Model file for the job. Use its own axes, mm. Face numbers are marked on the shaded views. Round coordinates to 2 decimals unless told otherwise and drop trailing zeros. Order: outer loops, then holes, each group sorted by start corner. A loop starts at its lowest first (then second) coordinate and runs counter-clockwise, first axis right, second up. Notation, with made-up numbers: (-30.5, 59.25) - (-9.5, 59.25) arc R12 ccw to (-9.5, 63.25) - close; hole circle Ø2 at (81.25, 63.5). An arc over 180 degrees is marked (long way). Write item = value, one per line. Start each with the question number.
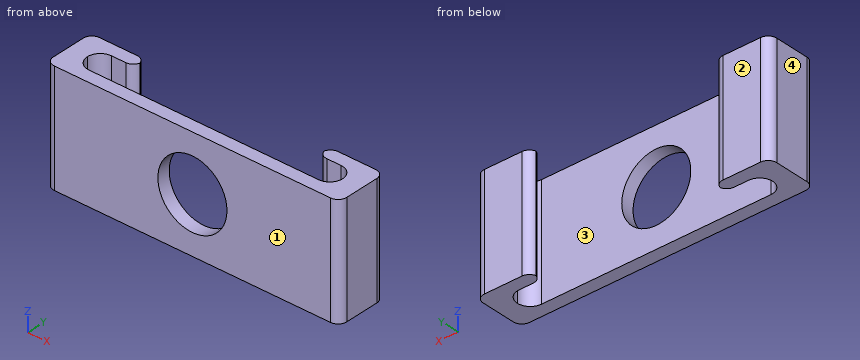
from build123d import *

# Parameters (mm, degrees)
F0_R        = 8
F1_DEPTH    = 12
F3_DEPTH    = 40
F4_T1_DEPTH = 36


# Not quite as in the source:
# - a fillet or chamfer that OpenCascade refuses, or shapes differently, is made with other operations: its cross-section is extruded or revolved along the edge and cut away or added
# - a feature names something its author has since deleted; it is built from what else it names


with BuildPart() as f1:
    # F0 (on Front) → F1 (new body)
    with BuildSketch(Plane.XZ):
        Polygon((34, 13), (-34, 13), (-34, 0), (-34, -13), (34, -13), align=None)
        Circle(F0_R, mode=Mode.SUBTRACT)
    extrude(amount=F1_DEPTH)

    # F2 (on face) → F3 (cut)
    with BuildSketch(Plane.XY.offset(13)):
        with BuildLine():
            Line((-21.2670322508, -3), (-26.5711637536, -3))
            ThreePointArc((-26.5711637536, -3), (-28.6924840972, -3.8786796564), (-29.5711637536, -6))
            ThreePointArc((-29.5711637536, -6), (-28.6924840972, -8.1213203436), (-26.5711637536, -9))
            Line((-26.5711637536, -9), (26.5711637536, -9))
            ThreePointArc((26.5711637536, -9), (28.6924840972, -8.1213203436), (29.5711637536, -6))
            ThreePointArc((29.5711637536, -6), (28.6924840972, -3.8786796564), (26.5711637536, -3))
            Line((26.5711637536, -3), (21.2670322508, -3))
            Line((21.2670322508, -3), (21.2670322508, 0))
            Line((21.2670322508, 0), (0, 0))
            Line((0, 0), (-21.2670322508, 0))
            Line((-21.2670322508, 0), (-21.2670322508, -3))
        make_face()
    extrude(amount=-F3_DEPTH, mode=Mode.SUBTRACT)

    # F4: fillet of radius 2 on 8 edges, made by hand

    # F4_s2 → F4_t1 (cut)
    with BuildSketch(Plane.XY.offset(-18)):
        with BuildLine():
            ThreePointArc((32, -12), (33.4142135624, -11.4142135624), (34, -10))
            Line((34, -10), (34, -12))
            Line((34, -12), (32, -12))
        make_face()
        with BuildLine():
            ThreePointArc((32, 0), (33.4142135624, -0.5857864376), (34, -2))
            Line((34, -2), (34, 0))
            Line((34, 0), (32, 0))
        make_face()
        with BuildLine():
            ThreePointArc((-21.2670322508, -2), (-21.8528186884, -0.5857864376), (-23.2670322508, 0))
            Line((-23.2670322508, 0), (-21.2670322508, 0))
            Line((-21.2670322508, 0), (-21.2670322508, -2))
        make_face()
        with BuildLine():
            ThreePointArc((23.2670322508, 0), (21.8528186884, -0.5857864376), (21.2670322508, -2))
            Line((21.2670322508, -2), (21.2670322508, 0))
            Line((21.2670322508, 0), (23.2670322508, 0))
        make_face()
        with BuildLine():
            ThreePointArc((-32, 0), (-33.4142135624, -0.5857864376), (-34, -2))
            Line((-34, -2), (-34, 0))
            Line((-34, 0), (-32, 0))
        make_face()
        with BuildLine():
            ThreePointArc((-34, -10), (-33.4142135624, -11.4142135624), (-32, -12))
            Line((-32, -12), (-34, -12))
            Line((-34, -12), (-34, -10))
        make_face()
        with BuildLine():
            ThreePointArc((-23.2670322508, -3), (-21.8528186884, -2.4142135624), (-21.2670322508, -1))
            Line((-21.2670322508, -1), (-21.2670322508, -3))
            Line((-21.2670322508, -3), (-23.2670322508, -3))
        make_face()
        with BuildLine():
            ThreePointArc((21.2670322508, -1), (21.8528186884, -2.4142135624), (23.2670322508, -3))
            Line((23.2670322508, -3), (21.2670322508, -3))
            Line((21.2670322508, -3), (21.2670322508, -1))
        make_face()
    extrude(amount=F4_T1_DEPTH, mode=Mode.SUBTRACT)


solid = f1.part
Item 1: Drop flat-ended pins along their axis: pin 1 (4 mm diameter, centred on x = -17.5, z = -3.5, fed in from +Y); pin 2 (12 mm diameter, centred on x = 16, z = 3.5, fed in from +Y); pin 3 (2 mm diameter, centred on y = -1.5, z = -4.5, fed in from -X); pin 4 (2 mm diameter, centred on x = 2, y = -6.5, fed in from +Z). Give the stop position or say it passes through.
Item 2: Saw through at A-A, the plane x = 0. Give the cut face in (y, z).
Item 3: Saw through at C-C, the plane y = -5.25. Give the cut face in (x, z).
Item 4: Probe L1, parallel to X at y = -9.7, z = 0; L2, parallel to Z at x = 0, y = -9.85; L3, parallel to Y at x = 25, z = 8.5. List the from-to ranges inside material, lowest first.
Item 5: Saw through at B-B, the plane z = 0. Give the cut face in (x, y).
Item 6: Saw through at D-D, the plane z = -5.5. Give the cut face in (x, y), then the cut area to 3 significant figures.
Item 7: Mould opens along Y. For the marked faces 1, 2, 3 and 4 say: +Y half, -Y half, draft (parallel to the pull), parting line (faces both ways), or undercut.
Check sheet entries:
q1.pin_1 = -9
q1.pin_2 = -0.45
q1.pin_3 = -34
q1.pin_4 = through
q2.outline = (-12, -13) - (-9, -13) - (-9, -8) - (-12, -8) - close; (-12, 8) - (-9, 8) - (-9, 13) - (-12, 13) - close
q3.outline = (-34, -13) - (-29.48, -13) - (-29.48, 13) - (-34, 13) - close; (29.48, -13) - (34, -13) - (34, 13) - (29.48, 13) - close
q4.L1 = -34 to -8, 8 to 34
q4.L2 = -13 to -8, 8 to 13
q4.L3 = -12 to -9, -3 to 0
q5.outline = (-34, -10) arc R2 ccw to (-32, -12) - (-8, -12) - (-8, -9) - (-26.57, -9) arc R3 cw to (-26.57, -3) - (-23.27, -3) arc R2 ccw to (-21.33, -1.5) arc R2 ccw to (-23.27, 0) - (-32, 0) arc R2 ccw to (-34, -2) - close; (8, -12) - (32, -12) arc R2 ccw to (34, -10) - (34, -2) arc R2 ccw to (32, 0) - (23.27, 0) arc R2 ccw to (21.33, -1.5) arc R2 ccw to (23.27, -3) - (26.57, -3) arc R3 cw to (26.57, -9) - (8, -9) - close
q6.outline = (-34, -10) arc R2 ccw to (-32, -12) - (-5.81, -12) - (-5.81, -9) - (-26.57, -9) arc R3 cw to (-26.57, -3) - (-23.27, -3) arc R2 ccw to (-21.33, -1.5) arc R2 ccw to (-23.27, 0) - (-32, 0) arc R2 ccw to (-34, -2) - close; (5.81, -12) - (32, -12) arc R2 ccw to (34, -10) - (34, -2) arc R2 ccw to (32, 0) - (23.27, 0) arc R2 ccw to (21.33, -1.5) arc R2 ccw to (23.27, -3) - (26.57, -3) arc R3 cw to (26.57, -9) - (5.81, -9) - close
q6.area = 300 mm2
q7.face_1 = -Y half
q7.face_2 = +Y half
q7.face_3 = undercut
q7.face_4 = draft
